```python
from build123d import *

# Parameters (mm, degrees)
SKETCH1_R           = 1.6
BOSS_EXTRUDE1_DEPTH = 3
CHAMFER1_SIZE       = 0.5


with BuildPart() as part:
    # Sketch1 → Boss-Extrude1 (new, symmetric)
    with BuildSketch(Plane(origin=(0, 0, 0), x_dir=(1, 0, 0), z_dir=(0, 1, 0))):
        with BuildLine():
            Line((0, 7.5), (120, 7.5))
            ThreePointArc((120, 7.5), (127.5, 0), (120, -7.5))
            Line((120, -7.5), (0, -7.5))
            ThreePointArc((0, -7.5), (-7.5, 0), (0, 7.5))
        make_face()
        with Locations(Location((0, 0, 0), (0, 0, 270))):
            Circle(SKETCH1_R, mode=Mode.SUBTRACT)
        with Locations(Location((120, 0, 0), (0, 0, 270))):
            Circle(SKETCH1_R, mode=Mode.SUBTRACT)
        with Locations(Location((24.5, 0, 0), (0, 0, 270))):
            Circle(SKETCH1_R, mode=Mode.SUBTRACT)
        with Locations(Location((95.5, 0, 0), (0, 0, 270))):
            Circle(SKETCH1_R, mode=Mode.SUBTRACT)
    extrude(amount=BOSS_EXTRUDE1_DEPTH, both=True)

    # Chamfer1
    chamfer1_edges = [part.edges().sort_by_distance(p)[0] for p in [
        (95.5, 3, -1.6),
        (-7.5, -3, 0),
        (60, -3, -7.5),
        (127.5, -3, 0),
        (60, -3, 7.5),
        (120, -3, -1.6),
        (0, -3, -1.6),
        (24.5, -3, -1.6),
        (95.5, -3, -1.6),
        (24.5, 3, -1.6),
        (0, 3, -1.6),
        (120, 3, -1.6),
        (60, 3, 7.5),
        (127.5, 3, 0),
        (60, 3, -7.5),
        (-7.5, 3, 0),
    ]]
    chamfer(chamfer1_edges, length=CHAMFER1_SIZE)


solid = part.part
```
Geometry check sheet. Reference: the model listing, model coordinates, mm. Give positions to 0.01 mm unless a question says otherwise; leave off trailing zeros. Loops run counter-clockwise (first coordinate to the right, second up) from the corner with the lowest first, then second, coordinate; pieces in that order, holes last. Notation, with made-up numbers: M 37,-8.5 L 52,-8.5 A34 cw 52,22.5 Z; hole C 40.25,34.5 d8. An arc over 180 degrees is marked long. Write item = value, one per line.
(1) Sectioned sample at C-C, the plane z = 0. State how many separate pieces and enclosed holes the cut face has, plus the area to 3 significant figures.
Answer below:
separate_pieces = 5
enclosed_holes = 0
area = 731 mm2
(2) Release check for a two-part mould opening along Z. For faces 1 (the face through (-7.5, 0.04, 0.16)), 2 (the face through (61, 0, 7.5)), 3 (the face through (-0.97, -0.04, -1.27)) record: released by +Z, released by -Z, zero draft, split by the parting line, or undercut.
Answer below:
face_1 = split by the parting line
face_2 = released by +Z
face_3 = undercut
(3) Material ranges on line 1 (X direction, y = -0.65, z = 0); line 2 (Z direction, x = 95.5, y = -0.5); line 3 (Z direction, x = 96, y = 0.75), recorded low to high. Write a range as [from, to].
Answer below:
line_1 = [-7.5, -1.6], [1.6, 22.9], [26.1, 93.9], [97.1, 118.4], [121.6, 127.5]
line_2 = [-7.5, -1.6], [1.6, 7.5]
line_3 = [-7.5, -1.52], [1.52, 7.5]
(4) Sectioned sample at A-A, the plane x = 24.5. Record the cut outline in (y, z).
Answer below:
outline = M -3,-7 L -2.5,-7.5 L 2.5,-7.5 L 3,-7 L 3,-2.1 L 2.5,-1.6 L -2.5,-1.6 L -3,-2.1 Z; M -3,2.1 L -2.5,1.6 L 2.5,1.6 L 3,2.1 L 3,7 L 2.5,7.5 L -2.5,7.5 L -3,7 Z
(5) Sectioned sample at B-B, the plane y = 0. Record the cut outline in (x, z), plus the area to 3 significant figures.
Answer below:
outline = M 0,-7.5 L 120,-7.5 A7.5 ccw 120,7.5 L 0,7.5 A7.5 ccw Z; hole C 0,0 d3.2; hole C 24.5,0 d3.2; hole C 95.5,0 d3.2; hole C 120,0 d3.2
area = 1,940 mm2
